Check sheet for the modelled part. Datum: model origin and axes. Units: mm. Face numbers are marked on the shaded views. Round coordinates to 2 decimals unless told otherwise and drop trailing zeros. Loops run counter-clockwise (first coordinate to the right, second up) from the corner with the lowest first, then second, coordinate; pieces in that order, holes last. Notation, with made-up numbers: (-19.75, 65) - (23.25, 65) arc R30 ccw to (23.25, 92) - close; hole circle Ø1 at (-26, 66). An arc over 180 degrees is marked (long way). Put each result on its own line as item: value. Start each with the question number.
Item 1: Section check B-B, the plane z = -32.5. Record the cut outline in (x, y), and give its area (3 significant figures).
Item 2: Section check C-C, the plane x = -7.5. Record the cut outline in (y, z), and give its area (3 significant figures).
Item 3: Material ranges on line 1 along Y through (x, z) = (1.55, -32.5); line 2 along Y through (x, z) = (2, -32); line 3 along Z through (x, y) = (1.5, 19), recorded low to high.
Item 4: Section check A-A, the plane z = 18. Record the cut outline in (x, y), and give its area (3 significant figures).
Item 5: Gauge pin test, flat ends, axial feed: pin 1 Ø2.5 at (x, z) = (-14, 52.5) entering from +Y; pin 2 Ø12 at (x, y) = (-25, -42) entering from +Z; pin 3 Ø10 at (y, z) = (-29, -48.5) entering from -X; pin 4 Ø2.5 at (y, z) = (52.5, -32.5) entering from -X. Record the tip position at first contact, or that the pin passes through.
Item 6: Draft check along Y on the marked faces 1 and 2. Enter one of: pulls with the +Y half, pulls with the -Y half, needs draft (parallel to the pull), parting line crosses it, or undercut.
Item 7: Section check D-D, the plane y = 52.5. Record the cut outline in (x, z), and give its area (3 significant figures).
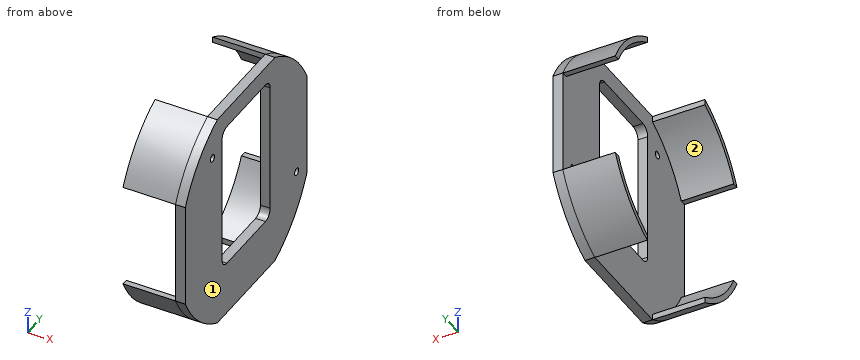
from build123d import *
from build123d.topology import SkipClean

# Parameters (mm, degrees)
SKETCH_1_R          = 70
SKETCH_1_R_2        = 2.1
SKETCH_1_W          = 85
SKETCH_1_H          = 50
EXTRUDE_2_DEPTH     = 5.6
FILLET_1_R          = 5
EXTRUDE_START       = 30
EXTRUDE_3_DEPTH     = 30
CUT_EXTRUDE_1_DEPTH = 111.453610172


with BuildPart() as part:
    # ｽｹｯﾁ1 → ﾎﾞｽ - 押し出し2 (new body)
    with BuildSketch(Plane(origin=(0, 0, 0), x_dir=(0, 0, -1), z_dir=(1, 0, 0))):
        with Locations((10, 0)):
            Circle(SKETCH_1_R)
        with Locations(Location((32.5, 52.5, 0), (0, 0, 180))):
            Circle(SKETCH_1_R_2, mode=Mode.SUBTRACT)
        with Locations((-32.5, -35)):
            Circle(SKETCH_1_R_2, mode=Mode.SUBTRACT)
        Rectangle(SKETCH_1_W, SKETCH_1_H, mode=Mode.SUBTRACT)
    extrude(amount=EXTRUDE_2_DEPTH)

    # ﾌｨﾚｯﾄ1
    fillet_1_edges = [part.edges().sort_by_distance(p)[0] for p in [
        (2.8, -25, -42.5),
        (2.8, 25, -42.5),
        (2.8, 25, 42.5),
        (2.8, -25, 42.5),
    ]]
    fillet(fillet_1_edges, radius=FILLET_1_R)

    # ｽｹｯﾁ2 → ﾎﾞｽ - 押し出し3 (add)
    with SkipClean():  # the faces are left unmerged after this step: merging them gives an invalid solid
        with BuildSketch(Plane.ZY.offset(EXTRUDE_START)):
            with BuildLine():
                ThreePointArc((-40, 63.245553203), (-59.497474683, 49.497474683), (-73.245553203, 30))
                Line((-73.245553203, 30), (-69.908263203, 30))
                ThreePointArc((-69.908263203, 30), (-57.376154339, 47.376154339), (-40, 59.908263203))
                Line((-40, 59.908263203), (-40, 63.245553203))
            make_face()
            with BuildLine():
                ThreePointArc((53.245553203, 30), (39.497474683, 49.497474683), (20, 63.245553203))
                Line((20, 63.245553203), (20, 59.908263203))
                ThreePointArc((20, 59.908263203), (37.376154339, 47.37615434), (49.908263203, 30))
                Line((49.908263203, 30), (53.245553203, 30))
            make_face()
            with BuildLine():
                Line((-69.908263203, -30), (-73.245553203, -30))
                ThreePointArc((-73.245553203, -30), (-59.497474683, -49.497474683), (-40, -63.245553203))
                Line((-40, -63.245553203), (-40, -59.908263203))
                ThreePointArc((-40, -59.908263203), (-57.376154339, -47.376154339), (-69.908263203, -30))
            make_face()
            with BuildLine():
                Line((20, -59.908263203), (20, -63.245553203))
                ThreePointArc((20, -63.245553203), (39.497474683, -49.497474683), (53.245553203, -30))
                Line((53.245553203, -30), (49.908263203, -30))
                ThreePointArc((49.908263203, -30), (37.376154339, -47.37615434), (20, -59.908263203))
            make_face()
        extrude(amount=-EXTRUDE_3_DEPTH)

    # ｽｹｯﾁ3 → ｶｯﾄ - 押し出し1 (cut, through all)
    with BuildSketch(Plane.ZY):
        with BuildLine():
            Line((20, 63.245553203), (-40, 63.245553203))
            ThreePointArc((-40, 63.245553203), (-10, 70), (20, 63.245553203))
        make_face()
        with BuildLine():
            Line((-73.245553203, 30), (-73.245553203, -30))
            ThreePointArc((-73.245553203, -30), (-80, 0), (-73.245553203, 30))
        make_face()
        with BuildLine():
            Line((-40, -63.245553203), (20, -63.245553203))
            ThreePointArc((20, -63.245553203), (-10, -70), (-40, -63.245553203))
        make_face()
        with BuildLine():
            Line((53.245553203, -30), (53.245553203, 30))
            ThreePointArc((53.245553203, 30), (60, 0), (53.245553203, -30))
        make_face()
    extrude(amount=-CUT_EXTRUDE_1_DEPTH, mode=Mode.SUBTRACT)


solid = part.part
Check result:
1. outline: (0, -63.25) - (5.6, -63.25) - (5.6, -25) - (0, -25) - close; (0, 25) - (5.6, 25) - (5.6, 50.4) - (0, 50.4) - close; (0, 54.6) - (5.6, 54.6) - (5.6, 63.25) - (0, 63.25) - close
1. area: 405 mm²
2. outline: (-63.25, -40) arc R70 ccw to (-30, -73.25) - (-30, -69.91) arc R67 cw to (-59.91, -40) - close; (-63.25, 20) - (-59.91, 20) arc R67 cw to (-30, 49.91) - (-30, 53.25) arc R70 ccw to start; (30, -73.25) arc R70 ccw to (63.25, -40) - (59.91, -40) arc R67 cw to (30, -69.91) - close; (30, 49.91) arc R67 cw to (59.91, 20) - (63.25, 20) arc R70 ccw to (30, 53.25) - close
2. area: 546 mm²
3. line 1: -63.25 to -25, 25 to 50.4, 54.6 to 63.25
3. line 2: -63.25 to -25, 25 to 50.46, 54.54 to 63.25
3. line 3: -73.25 to -42.5, 42.5 to 53.25
4. outline: (0, -63.25) - (5.6, -63.25) - (5.6, -25) - (0, -25) - close; (0, 25) - (5.6, 25) - (5.6, 63.25) - (0, 63.25) - close
4. area: 428 mm²
5. pin 1: y = 33.89
5. pin 2: z = 50.03
5. pin 3: x = 0
5. pin 4: through
6. face 1: needs draft
6. face 2: undercut
7. outline: (-30, -56.3) - (5.6, -56.3) - (5.6, -34.6) - (0, -34.6) - (0, -51.63) - (-30, -51.63) - close; (-30, 31.63) - (0, 31.63) - (0, -30.4) - (5.6, -30.4) - (5.6, 36.3) - (-30, 36.3) - close
7. area: 776 mm²
